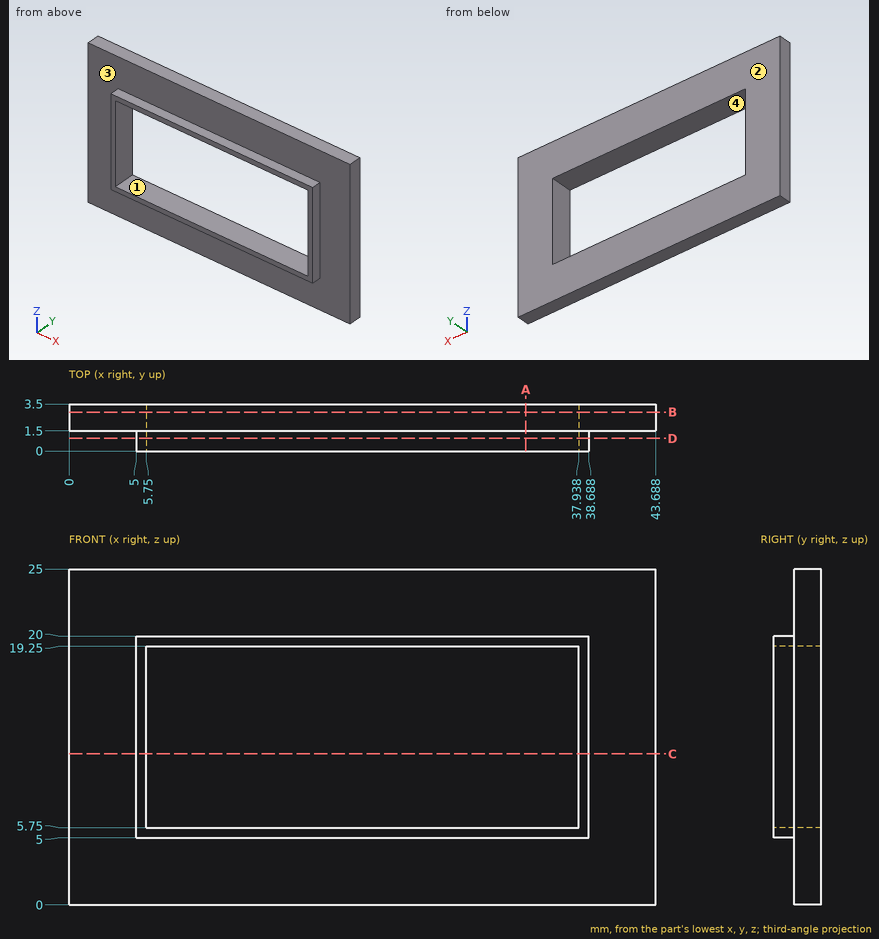
For this review, use the dimensioned drawing (mm, ordinates from the lowest corner) and the shaded views. A direction names the side the tool comes from. Round coordinates to 2 decimals unless told otherwise and drop trailing zeros. Loops run counter-clockwise (first coordinate to the right, second up) from the corner with the lowest first, then second, coordinate; pieces in that order, holes last. Notation, with made-up numbers: M 30,57 L 78,57 A16 ccw 78,81 Z; hole C 24.5,-12 d3. An arc over 180 degrees is marked long. Answer as CSV lines item,"result".
1. Insertion check: pin 1 Ø1.6 at (y, z) = (0.5, 13) entering from +X; pin 2 Ø0.8 at (y, z) = (1, 12.5) entering from -X; pin 3 Ø8 at (x, z) = (31, 11.5) entering from -Y (3 decimals); pin 4 Ø0.8 at (x, y) = (15, 0.5) entering from -Z. Each pin has a flat end and moves straight along its axis. Give the tip position at first contact, or say it passes through.
Outcome:
pin 1,"stops at x = 38.69"
pin 2,"stops at x = 5"
pin 3,"passes through"
pin 4,"stops at z = 5"
2. We need section D-D (y = 0.95). Give the boundary of the cut face in (x, z).
Outcome:
outline,"M 5,5 L 38.69,5 L 38.69,20 L 5,20 Z; hole M 5.75,5.75 L 37.94,5.75 L 37.94,19.25 L 5.75,19.25 Z"
3. For the marked faces 1 and 2, list the 3-axis set-ups (+Z, -Z, +X, -X, +Y, -Y) from which the entire face can be reached by the end or side of a thin tool; tool diameter is ignored.
Outcome:
face 1,"+Y, -Y"
face 2,"+Z, -Z, +X, -X, +Y"
4. Draft analysis for pull direction X (two halves, no side actions). For the marked faces 3 and 4, state which applies: pulls with the +X half, pulls with the -X half, needs draft (parallel to the pull), parting line crosses it, or undercut.
Outcome:
face 3,"needs draft"
face 4,"undercut"
5. To check wall thickness, follow L1, parallel to X at y = 2.6, z = 13; L2, parallel to Z at x = 21, y = 3.05; L3, parallel to X at y = 0.4, z = 8. State the ranges of each line that lie inside material, in increasing order. Write a range as [from, to].
Outcome:
L1,"x = [0, 5.75], [37.94, 43.69]"
L2,"z = [0, 5.75], [19.25, 25]"
L3,"x = [5, 5.75], [37.94, 38.69]"
6. We need section A-A (x = 34). Give the boundary of the cut face in (y, z), plus the area to 4 significant figures.
Outcome:
outline,"M 0,5 L 1.5,5 L 1.5,0 L 3.5,0 L 3.5,5.75 L 0,5.75 Z; M 0,19.25 L 3.5,19.25 L 3.5,25 L 1.5,25 L 1.5,20 L 0,20 Z"
area,"25.25 mm2"
7. We need section B-B (y = 2.9). Give the boundary of the cut face in (x, z), plus the area to 3 significant figures.
Outcome:
outline,"M 0,0 L 43.69,0 L 43.69,25 L 0,25 Z; hole M 5.75,5.75 L 37.94,5.75 L 37.94,19.25 L 5.75,19.25 Z"
area,"658 mm2"
8. We need section C-C (z = 11.25). Give the boundary of the cut face in (x, y).
Outcome:
outline,"M 0,1.5 L 5,1.5 L 5,0 L 5.75,0 L 5.75,3.5 L 0,3.5 Z; M 37.94,0 L 38.69,0 L 38.69,1.5 L 43.69,1.5 L 43.69,3.5 L 37.94,3.5 Z"
